Design review of the part built by this model. Coordinates are the model's own, in mm. A direction names the side the tool comes from. Coordinates: 2 decimals unless noted, no trailing zeros. Write each loop counter-clockwise with the first axis right and the second up, starting at its lowest first coordinate (ties: lowest second). Pieces come first, ordered by that corner, then holes. Notation, with made-up numbers: (-37.5, -18.5) - (-18.5, -18.5) arc R27 ccw to (-18.5, 11.5) - close; hole circle Ø10 at (82.25, 47.5). An arc over 180 degrees is marked (long way). One line per item, written item: value.
from build123d import *

# Parameters (mm, degrees)
F0_W     = 28
F0_H     = 12
F1_DEPTH = 30
F2_W     = 21.6
F2_H     = 23.6
F3_DEPTH = 10
F5_DEPTH = 24.8
F6_R     = 1


with BuildPart() as f1:
    # F0 (on Front) → F1 (new body)
    with BuildSketch(Plane.XZ):
        with Locations((14, 6)):
            Rectangle(F0_W, F0_H)
    extrude(amount=F1_DEPTH)

    # F2 (on face) → F3 (cut)
    with BuildSketch(Plane.XY.offset(12)):
        with Locations((14, -15)):
            Rectangle(F2_W, F2_H)
    extrude(amount=-F3_DEPTH, mode=Mode.SUBTRACT)

    # F4 (on face) → F5 (cut, through all)
    with BuildSketch(Plane(origin=(0, 0, 0), x_dir=(0, -1, 0), z_dir=(-1, 0, 0))):
        Polygon((3.2, 10.4), (1.6, 10.4), (1.6, 8.8), (3.2, 8.8), (15, 8.8), (26.8, 8.8), (28.4, 8.8), (28.4, 10.4), (26.8, 10.4), (26.8, 12), (3.2, 12), align=None)
    extrude(amount=-F5_DEPTH, mode=Mode.SUBTRACT)

    # F6
    f6_edges = [f1.edges().sort_by_distance(p)[0] for p in [
        (0, 0, 6),
        (14, 0, 12),
        (0, -30, 6),
        (14, -30, 12),
        (28, 0, 6),
        (28, -30, 6),
        (28, -15, 12),
    ]]
    fillet(f6_edges, radius=F6_R)


solid = f1.part
1. For faces 1 (the face through (12, -2, 10.4)), 2 (the face through (28, -15, 5)), 3 (the face through (12, -26.8, 11)), 4 (the face through (14, -15, 2)), list the 3-axis set-ups (+Z, -Z, +X, -X, +Y, -Y) from which the entire face can be reached by the end or side of a thin tool; tool diameter is ignored.
Answer block:
face 1: -X
face 2: +Z, -Z, +X, +Y, -Y
face 3: +Z, -X
face 4: +Z
2. Insertion check: pin 1 Ø0.5 at (x, z) = (16.5, 11.5) entering from -Y; pin 2 Ø7.5 at (x, y) = (14.5, -17.5) entering from +Z. Each pin has a flat end and moves straight along its axis. Give the tip position at first contact, or say it passes through.
Answer block:
pin 1: stops at y = -29.97
pin 2: stops at z = 2
3. Mouldability with a two-part tool opening along X and no side actions: class faces 5 (the face through (12, -28.4, 10)), 6 (the face through (0.285, -0.301, 6.084)), 7 (the face through (3.2, -15, 5)) as released by +X, released by -X, zero draft, split by the parting line, or undercut.
Answer block:
face 5: zero draft
face 6: released by -X
face 7: undercut
4. Consider section B-B, the plane y = -2.5. Write out the cut boundary in (x, z), then the cut area to 3 significant figures.
Answer block:
outline: (0, 0) - (28, 0) - (28, 11) arc R1 ccw to (27, 12) - (0, 12) - (0, 10.4) - (24.8, 10.4) - (24.8, 8.8) - (0, 8.8) - close
area: 296 mm^2
5. Wall thickness on line 1 along Y through (x, z) = (24, 4.25); line 2 along X through (y, z) = (-18, 5.5); line 3 along Z through (x, y) = (23.5, -9): over which ranges is each line inside the solid? List them lowest first.
Answer block:
line 1: y = -30 to -26.8, -3.2 to 0
line 2: x = 0 to 3.2, 24.8 to 28
line 3: z = 0 to 2
6. Consider section C-C, the plane z = 9.75. Write out the cut boundary in (x, y).
Answer block:
outline: (0, -29) arc R1 ccw to (1, -30) - (27, -30) arc R1 ccw to (28, -29) - (28, -1) arc R1 ccw to (27, 0) - (1, 0) arc R1 ccw to (0, -1) - (0, -1.6) - (24.8, -1.6) - (24.8, -28.4) - (0, -28.4) - close
7. Consider section A-A, the plane z = 5.25. Write out the cut boundary in (x, y).
Answer block:
outline: (0, -29) arc R1 ccw to (1, -30) - (27, -30) arc R1 ccw to (28, -29) - (28, -1) arc R1 ccw to (27, 0) - (1, 0) arc R1 ccw to (0, -1) - close; hole (3.2, -26.8) - (24.8, -26.8) - (24.8, -3.2) - (3.2, -3.2) - close
8. Consider section D-D, the plane x = 21. Write out the cut boundary in (y, z).
Answer block:
outline: (-30, 0) - (0, 0) - (0, 11) arc R1 ccw to (-1, 12) - (-3.2, 12) - (-3.2, 10.4) - (-1.6, 10.4) - (-1.6, 8.8) - (-3.2, 8.8) - (-3.2, 2) - (-26.8, 2) - (-26.8, 8.8) - (-28.4, 8.8) - (-28.4, 10.4) - (-26.8, 10.4) - (-26.8, 12) - (-29, 12) arc R1 ccw to (-30, 11) - close
